from build123d import *

# Parameters (mm, degrees)
PAD_DEPTH            = 22
SKETCH001_R          = 3.1
SKETCH001_R_2        = 0.5
POCKET_DEPTH         = 5.001
POCKET_DEPTH_BACK    = -27.001
SKETCH002_R          = 3.1
POCKET001_DEPTH      = 5
SKETCH003_R          = 1.6
POCKET002_DEPTH      = 22.001
POCKET002_DEPTH_BACK = -22.001
SKETCH004_R          = 3
POCKET003_DEPTH      = 5
POCKET004_DEPTH      = 2.3
FILLET_R             = 1


with BuildPart() as part:
    # Sketch → Pad (new body, symmetric)
    with BuildSketch(Plane.XZ):
        Polygon((0, 27), (0, 0), (27, 0), (27, -5), (-32, -5), (-32, 7), (-5, 7), (-5, 27), align=None)
    extrude(amount=PAD_DEPTH, both=True)

    # Sketch001 → Pocket (cut, two sides)
    with BuildSketch(Plane.XY) as pocket_sk:
        with Locations((15, 12.5)):
            Circle(SKETCH001_R)
        with Locations((15, -12.5)):
            Circle(SKETCH001_R)
        with Locations((27, 0)):
            Circle(SKETCH001_R_2)
        with BuildLine():
            ThreePointArc((-16.803848, -3), (-26.859933, 3.518672), (-17.527864, -4))
            Line((-6, -4), (-17.527864, -4))
            Line((-6, -4), (-6, -10))
            Line((-6, -10), (-22, -10))
            ThreePointArc((-29.660444, 6.427876), (-31.063078, -4.226183), (-22, -10))
            Line((-18.392302, 19.856726), (-29.660444, 6.427876))
            ThreePointArc((-13.796055, 22), (-16.331753, 21.437843), (-18.392302, 19.856726))
            Line((-13.796055, 22), (-13.796055, 28.799225))
            Line((-13.796055, 28.799225), (-40.339119, 28.799225))
            Line((-40.339119, 28.799225), (-40.339119, -28.958258))
            Line((-40.339119, -28.958258), (-5, -28.958258))
            Line((-5, -28.958258), (-5, -3))
            Line((-16.803848, -3), (-5, -3))
        make_face()
    extrude(amount=-POCKET_DEPTH, mode=Mode.SUBTRACT)
    extrude(pocket_sk.sketch, amount=-POCKET_DEPTH_BACK, mode=Mode.SUBTRACT)

    # Sketch002 → Pocket001 (cut)
    with BuildSketch(Plane.YZ):
        with Locations((-12.5, 15)):
            Circle(SKETCH002_R)
        with Locations((12.5, 15)):
            Circle(SKETCH002_R)
    extrude(amount=-POCKET001_DEPTH, mode=Mode.SUBTRACT)

    # Sketch003 → Pocket002 (cut, two sides)
    with BuildSketch(Plane.XZ) as pocket002_sk:
        with Locations((-11, 1)):
            Circle(SKETCH003_R)
    extrude(amount=-POCKET002_DEPTH, mode=Mode.SUBTRACT)
    extrude(pocket002_sk.sketch, amount=-POCKET002_DEPTH_BACK, mode=Mode.SUBTRACT)

    # Sketch004 (on Face5 of Pocket002) → Pocket003 (cut)
    with BuildSketch(Plane(origin=(0, 22, 0), x_dir=(1, 0, 0), z_dir=(0, 1, 0))):
        with Locations((-11, -1)):
            Circle(SKETCH004_R)
    extrude(amount=-POCKET003_DEPTH, mode=Mode.SUBTRACT)

    # Sketch005 (on Face11 of Pocket003) → Pocket004 (cut)
    with BuildSketch(Plane.XZ.offset(10)):
        Polygon((-8.25, -0.587713), (-8.25, 2.587713), (-11, 4.175426), (-13.75, 2.587713), (-13.75, -0.587713), (-11, -2.175426), align=None)
    extrude(amount=-POCKET004_DEPTH, mode=Mode.SUBTRACT)

    # Fillet
    fillet_edges = [part.edges().sort_by_distance(p)[0] for p in [
        (27, -22, -2.5),
        (27, 22, -2.5),
        (-5, -22, 11),
        (-5, 22, 17),
    ]]
    fillet(fillet_edges, radius=FILLET_R)


solid = part.part
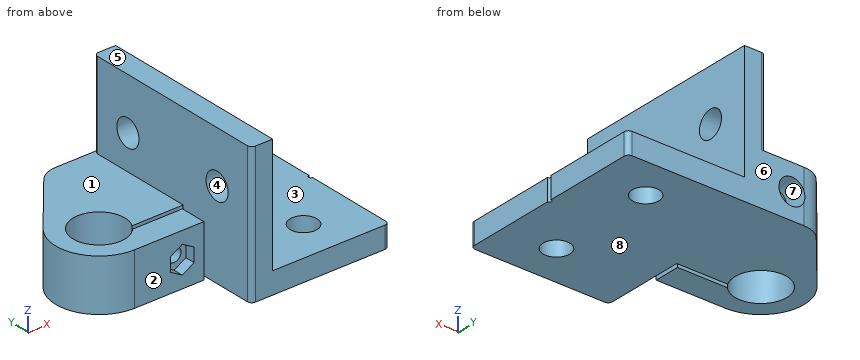
Work out the finished part from the listing and answer in its coordinate system (mm). Face numbers are marked on the shaded views. A direction names the side the tool comes from. Coordinates: 2 decimals unless noted, no trailing zeros. Loops run counter-clockwise (first coordinate to the right, second up) from the corner with the lowest first, then second, coordinate; pieces in that order, holes last. Notation, with made-up numbers: M 29,6.25 L 80,6.25 A25 ccw 80,28.25 Z; hole C 7.25,88 d2. An arc over 180 degrees is marked long. Answer in a Markdown table with one row per item. Add a question column.
1. Find section D-D, the plane z = 1. Write down the section's boundary in (x, y), then the cut area to 3 significant figures.
2. A tool of negligible diameter and unlimited length cuts with its end or side. For the marked faces 1, 2, 3, 4 and 5, from which of +Z, -Z, +X, -X, +Y, -Y can it reach the whole face along a straight path? Write none if from no direction.
3. Flat-ended cylindrical pins translate along their axes: P1, Ø5, axis at y = 11.5, z = 13.5, coming from the +X side; P2, Ø3.5, axis at x = -9, z = -0.5, coming from the -Y side; P3, Ø8, axis at y = 4, z = -0.5, coming from the -X side; P4, Ø4, axis at x = -14, y = 11, coming from the +Z side. Find the tip coordinate at first contact, or state that the pin passes through.
4. Find section A-A, the plane x = 15. Write down the section's boundary in (y, z), then the cut area to 3 significant figures.
5. Consider L1, parallel to X at y = -8, z = -0.5; L2, parallel to Y at x = 15, z = -2; L3, parallel to Z at x = -1.8, y = -12.5. Determine where each line is inside the solid, lowest interval first.
6. Find section C-C, the plane y = 3.5. Write down the section's boundary in (x, z).
7. The mould has two halves that part along Z. Classify the marked faces 6, 7 and 8: pulls with the +Z half, pulls with the -Z half, needs draft (parallel to the pull), parting line crosses it, or undercut.
8. Find section B-B, the plane z = 15. Write down the section's boundary in (x, y), then the cut area to 3 significant figures.
Reported:
| question | item | result |
|---|---|---|
| 1 | outline | M -29.66,6.43 A10 ccw -22,-10 L -13.75,-10 L -13.75,-7.7 L -12.6,-7.7 L -12.6,-4 L -17.53,-4 A6 cw long -16.8,-3 L -12.6,-3 L -12.6,17 L -14,17 L -14,22 A6 ccw -18.39,19.86 Z; M -9.4,-7.7 L -8.25,-7.7 L -8.25,-10 L -6,-10 L -6,-4 L -9.4,-4 Z; M -9.4,-3 L -5,-3 L -5,-21 A1 ccw -4,-22 L 0,-22 L 0,22 L -8,22 L -8,17 L -9.4,17 Z |
| 1 | area | 669 mm^2 |
| 2 | face 1 | +Z, -X, +Y, -Y |
| 2 | face 2 | +Z, -Z, -X, -Y |
| 2 | face 3 | +Z, +X, +Y, -Y |
| 2 | face 4 | +X, -X |
| 2 | face 5 | +Z, +X, -X, +Y, -Y |
| 3 | P1 | stops at x = 0 |
| 3 | P2 | stops at y = -10 |
| 3 | P3 | stops at x = -32 |
| 3 | P4 | stops at z = 7 |
| 4 | outline | M -22,-5 L -15.6,-5 L -15.6,0 L -22,0 Z; M -9.4,-5 L 9.4,-5 L 9.4,0 L -9.4,0 Z; M 15.6,-5 L 22,-5 L 22,0 L 15.6,0 Z |
| 4 | area | 158 mm^2 |
| 5 | L1 | x = -28 to -13.75, -8.25 to -6, -5 to 27 |
| 5 | L2 | y = -22 to -15.6, -9.4 to 9.4, 15.6 to 22 |
| 5 | L3 | z = -5 to 11.9, 18.1 to 27 |
| 6 | outline | M -31.37,-5 L -26.87,-5 L -26.87,7 L -31.37,7 Z; M -17.13,-5 L 27,-5 L 27,0 L 0,0 L 0,27 L -5,27 L -5,7 L -17.13,7 Z; hole C -11,1 d3.2 |
| 7 | face 6 | needs draft |
| 7 | face 7 | undercut |
| 7 | face 8 | pulls with the -Z half |
| 8 | outline | M -5,-21 A1 ccw -4,-22 L 0,-22 L 0,-15.6 L -5,-15.6 Z; M -5,-9.4 L 0,-9.4 L 0,9.4 L -5,9.4 Z; M -5,15.6 L 0,15.6 L 0,22 L -4,22 A1 ccw -5,21 Z |
| 8 | area | 158 mm^2 |
